from build123d import *

# Parameters (mm, degrees)
SKETCH_1_W          = 132
SKETCH_1_H          = 80
EXTRUDE_1_DEPTH     = 210
SKETCH_2_W          = 124
SKETCH_2_H          = 206
CUT_EXTRUDE_1_DEPTH = 76
SKETCH_3_R          = 13
SKETCH_3_R_2        = 3
CUT_EXTRUDE_2_DEPTH = 10
SKETCH_4_R          = 3.25
SKETCH_4_R_2        = 30
CUT_EXTRUDE_3_DEPTH = 10
FILLET_1_R          = 3


with BuildPart() as part:
    # 草图1 → 凸台-拉伸1 (new body)
    with BuildSketch(Plane.XY):
        Rectangle(SKETCH_1_W, SKETCH_1_H)
    extrude(amount=-EXTRUDE_1_DEPTH)

    # 草图2 → 切除-拉伸1 (cut)
    with BuildSketch(Plane(origin=(0, 40, 0), x_dir=(1, 0, 0), z_dir=(0, 1, 0))):
        with Locations((0, 107)):
            Rectangle(SKETCH_2_W, SKETCH_2_H)
    extrude(amount=-CUT_EXTRUDE_1_DEPTH, mode=Mode.SUBTRACT)

    # 草图3 → 切除-拉伸2 (cut)
    with BuildSketch(Plane.XY):
        with Locations((0, 15.5)):
            Circle(SKETCH_3_R)
        with Locations((-28, 15.5)):
            Circle(SKETCH_3_R_2)
        with Locations((28, 15.5)):
            Circle(SKETCH_3_R_2)
    extrude(amount=-CUT_EXTRUDE_2_DEPTH, mode=Mode.SUBTRACT)

    # 草图4 → 切除-拉伸3 (cut)
    with BuildSketch(Plane(origin=(0, -36, 0), x_dir=(1, 0, 0), z_dir=(0, 1, 0))):
        with Locations((26.516504294, 176.516504294)):
            Circle(SKETCH_4_R)
        with Locations((26.516504294, 123.483495706)):
            Circle(SKETCH_4_R)
        with Locations((-26.516504294, 123.483495706)):
            Circle(SKETCH_4_R)
        with Locations((-26.516504294, 176.516504294)):
            Circle(SKETCH_4_R)
        with Locations((0, 150)):
            Circle(SKETCH_4_R_2)
    extrude(amount=-CUT_EXTRUDE_3_DEPTH, mode=Mode.SUBTRACT)

    # 圆角1
    fillet_1_edges = [part.edges().sort_by_distance(p)[0] for p in [
        (-62, 2, -4),
        (62, 2, -4),
    ]]
    fillet(fillet_1_edges, radius=FILLET_1_R)


solid = part.part
Can you work these out from the model? Positions are in its coordinate system, mm. A direction names the side the tool comes from. Coordinates: 2 decimals unless noted, no trailing zeros. Order: outer loops, then holes, each group sorted by start corner. A loop starts at its lowest first (then second) coordinate and runs counter-clockwise, first axis right, second up. Notation, with made-up numbers: (-24, -14.75) - (30, -14.75) arc R23 ccw to (30, 8.25) - close; hole circle Ø1 at (52.25, 55). An arc over 180 degrees is marked (long way). Answer as a JSON object with one key per item and string values. Group by question number.
Q1. Imagine slicing it at D-D (z = -61). Please give me the cut outline in (x, y).
Q2. Will these pins go through, and if not, where does the flat tip stop? P1, Ø4, axis at x = 26.5, y = -18.5, coming from the -Z side; P2, Ø8.5, axis at x = 26.52, z = -176.52, coming from the +Y side.
Q3. We'd pull the mould along Z, two halves only. Please class faces 3 (the face through (25.812, -37.972, -173.344)), 4 (the face through (-1, 1, 0)), 5 (the face through (-62, 3, -107)), 6 (the face through (0, -38, -210)): +Z half, -Z half, draft (parallel to the pull), parting line (faces both ways), or undercut.
Q4. I need wall thicknesses on line 1 (X direction, y = 6, z = -15.5); line 2 (Y direction, x = 0, z = -1.9); line 3 (Y direction, x = -28, z = -1). Which ranges of each line are inside material? Lowest first, please. Write a range as from..to.
Q5. Imagine slicing it at B-B (y = 15.5). Please give me the cut outline in (x, z).
Q6. On a 3-axis mill with a long thin cutter (end or side, diameter ignored), from which of +Z, -Z, +X, -X, +Y, -Y can I reach the whole of each face in a straight line? I mean faces 1 (the face through (-6.503, -37.972, -120.713)), 2 (the face through (-1, -36, -108)). Say none if no direction works.
Q7. Imagine slicing it at C-C (x = 0). Please give me the cut outline in (y, z).
Q8. Imagine slicing it at A-A (z = -150). Please give me the cut outline in (x, y).
Determined:
{
 "1": {"outline": "(-66, -40) - (66, -40) - (66, 40) - (62, 40) - (62, -36) - (-62, -36) - (-62, 40) - (-66, 40) - close"},
 "2": {"P1": "stops at z = -4", "P2": "stops at y = -36"},
 "3": {"face 3": "undercut", "face 4": "+Z half", "face 5": "draft", "face 6": "-Z half"},
 "4": {"line 1": "x = -66..-62, 62..66", "line 2": "y = -40..2.5, 28.5..40", "line 3": "y = -40..12.5, 18.5..40"},
 "5": {"outline": "(-66, -210) - (-62, -210) - (-62, -7) arc R3 cw to (-59, -4) - (-31, -4) - (-31, 0) - (-66, 0) - close; (-25, -4) - (-13, -4) - (-13, 0) - (-25, 0) - close; (13, -4) - (25, -4) - (25, 0) - (13, 0) - close; (31, -4) - (59, -4) arc R3 cw to (62, -7) - (62, -210) - (66, -210) - (66, 0) - (31, 0) - close"},
 "6": {"face 1": "+Y, -Y", "face 2": "-Z, +Y"},
 "7": {"outline": "(-40, -210) - (-36, -210) - (-36, -180) - (-40, -180) - close; (-40, -120) - (-36, -120) - (-36, -4) - (2.5, -4) - (2.5, 0) - (-40, 0) - close; (28.5, -4) - (40, -4) - (40, 0) - (28.5, 0) - close"},
 "8": {"outline": "(-66, -40) - (-30, -40) - (-30, -36) - (-62, -36) - (-62, 40) - (-66, 40) - close; (30, -40) - (66, -40) - (66, 40) - (62, 40) - (62, -36) - (30, -36) - close"}
}
